```python
from build123d import *

# Parameters (mm, degrees)
EXTRUDE_THIN1_DEPTH = 7
BOSS_EXTRUDE1_DEPTH = 2
SKETCH3_R           = 7.55
SKETCH3_R_2         = 6.05
EXTRUDE_THIN2_DEPTH = 5
FILLET1_R           = 5
SKETCH4_W           = 1
SKETCH4_H           = 9.419182822
CUT_EXTRUDE1_DEPTH  = 818.680940253


with BuildPart() as part:
    # Sketch1 → Extrude-Thin1 (new body)
    with BuildSketch(Plane.XY):
        with BuildLine():
            Line((122.537316884, 771.044811258), (122.537316884, 739.044811258))
            ThreePointArc((122.537316884, 739.044811258), (127.955841432, 725.963335806), (141.037316884, 720.544811258))
            Line((141.037316884, 720.544811258), (194.037316884, 720.544811258))
            ThreePointArc((194.037316884, 720.544811258), (207.118792336, 725.963335806), (212.537316884, 739.044811258))
            Line((212.537316884, 739.044811258), (212.537316884, 771.044811258))
            ThreePointArc((212.537316884, 771.044811258), (207.118792336, 784.12628671), (194.037316884, 789.544811258))
            Line((194.037316884, 789.544811258), (141.037316884, 789.544811258))
            ThreePointArc((141.037316884, 789.544811258), (127.955841432, 784.12628671), (122.537316884, 771.044811258))
        make_face()
        with BuildLine():
            Line((124.037316884, 771.044811258), (124.037316884, 739.044811258))
            ThreePointArc((124.037316884, 739.044811258), (129.016501604, 727.023995978), (141.037316884, 722.044811258))
            Line((141.037316884, 722.044811258), (194.037316884, 722.044811258))
            ThreePointArc((194.037316884, 722.044811258), (206.058132165, 727.023995978), (211.037316884, 739.044811258))
            Line((211.037316884, 739.044811258), (211.037316884, 771.044811258))
            ThreePointArc((211.037316884, 771.044811258), (206.058132165, 783.065626538), (194.037316884, 788.044811258))
            Line((194.037316884, 788.044811258), (141.037316884, 788.044811258))
            ThreePointArc((141.037316884, 788.044811258), (129.016501604, 783.065626538), (124.037316884, 771.044811258))
        make_face(mode=Mode.SUBTRACT)
    extrude(amount=EXTRUDE_THIN1_DEPTH)

    # Sketch2 → Boss-Extrude1 (add)
    with BuildSketch(Plane.XY.offset(7)):
        with BuildLine():
            Line((122.537316884, 771.044811258), (122.537316884, 739.044811258))
            ThreePointArc((122.537316884, 739.044811258), (127.955841432, 725.963335806), (141.037316884, 720.544811258))
            Line((141.037316884, 720.544811258), (194.037316884, 720.544811258))
            ThreePointArc((194.037316884, 720.544811258), (207.118792336, 725.963335806), (212.537316884, 739.044811258))
            Line((212.537316884, 739.044811258), (212.537316884, 771.044811258))
            ThreePointArc((212.537316884, 771.044811258), (207.118792336, 784.12628671), (194.037316884, 789.544811258))
            Line((194.037316884, 789.544811258), (141.037316884, 789.544811258))
            ThreePointArc((141.037316884, 789.544811258), (127.955841432, 784.12628671), (122.537316884, 771.044811258))
        make_face()
    extrude(amount=BOSS_EXTRUDE1_DEPTH)

    # Sketch3 → Extrude-Thin2 (add)
    with BuildSketch(Plane(origin=(0, 0, 7), x_dir=(-1, 0, 0), z_dir=(0, 0, -1))):
        with Locations((-167.537316884, 739.044811258)):
            Circle(SKETCH3_R)
        with Locations((-167.537316884, 739.044811258)):
            Circle(SKETCH3_R_2, mode=Mode.SUBTRACT)
    extrude(amount=EXTRUDE_THIN2_DEPTH)

    # Fillet1
    fillet1_edges = [part.edges().sort_by_distance(p)[0] for p in [
        (175.087316884, 739.044811258, 7),
    ]]
    fillet(fillet1_edges, radius=FILLET1_R - 0.0001)  # a hair under: the kernel refuses the full size

    # Sketch4 → Cut-Extrude1 (cut, through all)
    with BuildSketch(Plane(origin=(0, 0, 7), x_dir=(-1, 0, 0), z_dir=(0, 0, -1))):
        with Locations((-170.834980474, 739.044811258)):
            Rectangle(SKETCH4_W, SKETCH4_H)
        with Locations((-167.834980474, 739.044811258)):
            Rectangle(SKETCH4_W, SKETCH4_H)
        with Locations((-164.834980474, 739.044811258)):
            Rectangle(SKETCH4_W, SKETCH4_H)
    extrude(amount=-CUT_EXTRUDE1_DEPTH, mode=Mode.SUBTRACT)


solid = part.part
```
Work out the finished part from the listing and answer in its coordinate system (mm). A direction names the side the tool comes from. Give positions to 0.01 mm unless a question says otherwise; leave off trailing zeros. Order: outer loops, then holes, each group sorted by start corner. A loop starts at its lowest first (then second) coordinate and runs counter-clockwise, first axis right, second up. Notation, with made-up numbers: (66.25, 53) - (78.25, 53) arc R37 cw to (78.25, 91) - close; hole circle Ø4 at (-14.5, 21). An arc over 180 degrees is marked (long way). One line per item, written item: value. Start each with the question number.
1. Which of the six approach directions +Z, -Z, +X, -X, +Y, -Y give full straight-line access (tool end or side, diameter ignored) to faces 1 (the face through (168.335, 739, 8)), 2 (the face through (166.5, 745.2, 2)), 3 (the face through (212.537, 755, 4))?
2. Section B-B, the plane x = 153 is taken. Write down the section's boundary in (y, z).
3. Section A-A, the plane z = 6 is taken. Write down the section's boundary in (x, y), then the cut area to 3 significant figures.
4. For a pull along Y with two mould halves and no side action, classify faces 4 (the face through (122.537, 755, 4)), 5 (the face through (124.037, 755, 3)), 6 (the face through (207.262, 783.982, 4.437)) as released by +Y, released by -Y, zero draft, split by the parting line, or undercut.
5. Section D-D, the plane z = 1 is taken. Write down the section's boundary in (x, y).
6. Each of these flat-tipped pins is pushed along its axis until it touches: pin 1 Ø2 at (x, z) = (199.5, 4.5) entering from +Y; pin 2 Ø4 at (x, y) = (180.5, 779) entering from -Z; pin 3 Ø2 at (y, z) = (737.5, 8) entering from +X. Where does it stop, or does it pass through?
7. Section C-C, the plane y = 753.5 is taken. Write down the section's boundary in (x, z).
8. Consider line 1 (X direction, y = 757, z = 5.5); line 2 (Y direction, x = 143.5, z = 6.5); line 3 (Z direction, x = 130, y = 732.5). Determine where each line is inside the solid, lowest interval first.
Filled sheet:
1. face 1: +Z, -Z
1. face 2: -Z
1. face 3: +Z, -Z, +X, +Y, -Y
2. outline: (720.54, 0) - (722.04, 0) - (722.04, 7) - (788.04, 7) - (788.04, 0) - (789.54, 0) - (789.54, 9) - (720.54, 9) - close
3. outline: (122.54, 739.04) arc R18.5 ccw to (141.04, 720.54) - (194.04, 720.54) arc R18.5 ccw to (212.54, 739.04) - (212.54, 771.04) arc R18.5 ccw to (194.04, 789.54) - (141.04, 789.54) arc R18.5 ccw to (122.54, 771.04) - close; circle Ø19.1 at (167.54, 739.04); hole (124.04, 739.04) arc R17 ccw to (141.04, 722.04) - (194.04, 722.04) arc R17 ccw to (211.04, 739.04) - (211.04, 771.04) arc R17 ccw to (194.04, 788.04) - (141.04, 788.04) arc R17 ccw to (124.04, 771.04) - close; hole circle Ø12.1 at (167.54, 739.04)
3. area: 594 mm²
4. face 4: zero draft
4. face 5: undercut
4. face 6: released by +Y
5. outline: (122.54, 739.04) arc R18.5 ccw to (141.04, 720.54) - (194.04, 720.54) arc R18.5 ccw to (212.54, 739.04) - (212.54, 771.04) arc R18.5 ccw to (194.04, 789.54) - (141.04, 789.54) arc R18.5 ccw to (122.54, 771.04) - close; hole (124.04, 739.04) arc R17 ccw to (141.04, 722.04) - (194.04, 722.04) arc R17 ccw to (211.04, 739.04) - (211.04, 771.04) arc R17 ccw to (194.04, 788.04) - (141.04, 788.04) arc R17 ccw to (124.04, 771.04) - close
6. pin 1: y = 789
6. pin 2: z = 7
6. pin 3: x = 212.53
7. outline: (122.54, 0) - (124.04, 0) - (124.04, 7) - (211.04, 7) - (211.04, 0) - (212.54, 0) - (212.54, 9) - (122.54, 9) - close
8. line 1: 122.54 to 124.04, 211.04 to 212.54
8. line 2: 720.54 to 722.04, 788.04 to 789.54
8. line 3: 7 to 9
